```python
from build123d import *

# Parameters (mm, degrees)
BOSS_EXTRUDE1_DEPTH = 16.6624
CUT_EXTRUDE1_REACH  = 42.603
SKETCH5_R           = 4.1656
CUT_EXTRUDE2_REACH  = 42.603
SKETCH6_R           = 4.1656
CUT_EXTRUDE9_REACH  = 47.74
SKETCH27_R          = 9.525
CUT_EXTRUDE10_REACH = 47.74
SKETCH28_R          = 9.525


with BuildPart() as part:
    # Sketch4 → Boss-Extrude1 (new, symmetric)
    with BuildSketch(Plane(origin=(0, 0, 0), x_dir=(0, 0, -1), z_dir=(1, 0, 0))):
        with BuildLine():
            Line((-19.05, -19.05), (19.05, -19.05))
            Line((19.05, -19.05), (19.05, 19.05))
            Line((19.05, 19.05), (15.330256, 19.05))
            ThreePointArc((15.330256, 19.05), (12.900216, 18.566635), (10.840128, 17.190128))
            Line((10.840128, 17.190128), (-17.190128, -10.840128))
            ThreePointArc((-17.190128, -10.840128), (-18.566635, -12.900216), (-19.05, -15.330256))
            Line((-19.05, -15.330256), (-19.05, -19.05))
        make_face()
        Polygon((-10.069744, -12.7), (12.7, -12.7), (12.7, 10.069744), align=None, mode=Mode.SUBTRACT)
    extrude(amount=BOSS_EXTRUDE1_DEPTH, both=True)

    # Sketch5 → Cut-Extrude1 (cut, up to next)
    with BuildSketch(Plane(origin=(0, -12.7, 0), x_dir=(1, 0, 0), z_dir=(0, 1, 0)), mode=Mode.PRIVATE) as cut_extrude1_sk1:
        with Locations(Location((0, 0, 0), (0, 0, 270))):
            Circle(SKETCH5_R)
    cut_extrude1_tool1 = extrude(cut_extrude1_sk1.sketch, amount=-CUT_EXTRUDE1_REACH, mode=Mode.PRIVATE) & part.part
    add(cut_extrude1_tool1.solids().sort_by_distance((0, -12.7, 0))[0], mode=Mode.SUBTRACT)

    # Sketch6 → Cut-Extrude2 (cut, up to next)
    with BuildSketch(Plane.XY.offset(-12.7), mode=Mode.PRIVATE) as cut_extrude2_sk1:
        Circle(SKETCH6_R)
    cut_extrude2_tool1 = extrude(cut_extrude2_sk1.sketch, amount=-CUT_EXTRUDE2_REACH, mode=Mode.PRIVATE) & part.part
    add(cut_extrude2_tool1.solids().sort_by_distance((0, 0, -12.7))[0], mode=Mode.SUBTRACT)

    # Cut-Extrude9: up to this plane
    cut_extrude9_end = Plane(origin=(16.6624, -12.7, 10.069744), z_dir=(0, -0.7071067811865474, -0.7071067811865477))
    # Sketch27 → Cut-Extrude9 (cut, up to the surface)
    with BuildSketch(Plane.XY.offset(19.05), mode=Mode.PRIVATE) as cut_extrude9_sk1:
        with Locations(Location((0, 0, 0), (0, 0, 270))):
            Circle(SKETCH27_R)
    cut_extrude9_tool1 = split(extrude(cut_extrude9_sk1.sketch, amount=-CUT_EXTRUDE9_REACH, mode=Mode.PRIVATE), bisect_by=cut_extrude9_end, keep=Keep.BOTH, mode=Mode.PRIVATE)
    add(cut_extrude9_tool1.solids().sort_by_distance((0, 0, 19.05))[0], mode=Mode.SUBTRACT)

    # Cut-Extrude10: up to this face of the body (flat: up to its plane)
    cut_extrude10_end = Plane(part.part.faces().sort_by_distance((-16.258791, -12.7, -1.315128))[0])
    # Sketch28 → Cut-Extrude10 (cut, up to the picked face)
    with BuildSketch(Plane(origin=(0, 19.05, 0), x_dir=(1, 0, 0), z_dir=(0, 1, 0)), mode=Mode.PRIVATE) as cut_extrude10_sk1:
        Circle(SKETCH28_R)
    cut_extrude10_tool1 = split(extrude(cut_extrude10_sk1.sketch, amount=-CUT_EXTRUDE10_REACH, mode=Mode.PRIVATE), bisect_by=cut_extrude10_end, keep=Keep.BOTH, mode=Mode.PRIVATE)
    add(cut_extrude10_tool1.solids().sort_by(Axis((0, 19.05, 0), (0, -1, 0)))[0], mode=Mode.SUBTRACT)


solid = part.part
```
Geometry check sheet. Reference: the model listing, model coordinates, mm. A direction names the side the tool comes from. Round coordinates to 2 decimals unless told otherwise and drop trailing zeros. Order: outer loops, then holes, each group sorted by start corner. A loop starts at its lowest first (then second) coordinate and runs counter-clockwise, first axis right, second up. Notation, with made-up numbers: (-14.75, -36.75) - (19.25, -36.75) arc R24 ccw to (19.25, -17.75) - close; hole circle Ø10 at (0.25, 5). An arc over 180 degrees is marked (long way). Use a Markdown table: item, result. Add a question column.
(1) Sectioned sample at C-C, the plane y = 2. Enter the section's corners in (x, z) (3 decimals), and give its area (3 significant figures).
(2) Sectioned sample at A-A, the plane x = -14. Enter the section's corners in (y, z), and give its area (3 significant figures).
(3) Material ranges on line 1 along Z through (x, y) = (-2.5, 6); line 2 along X through (y, z) = (9.5, -3.5), recorded low to high. Write a range as [from, to].
(4) Sectioned sample at B-B, the plane z = -8.5. Enter the section's corners in (x, y) (3 decimals).
(5) Depth check by flat-ended pin: pin 1 (5 mm diameter, centred on x = -0.5, y = 2.5, fed in from +Z); pin 2 (6 mm diameter, centred on x = 8.5, z = 0, fed in from +Y). Enter the tip coordinate at first touch or a pass-through.
(6) Sectioned sample at D-D, the plane x = 0. Enter the section's corners in (y, z) (3 decimals), and give its area (3 significant figures).
(7) Tool access check on faces 4 (the cylindrical face through (0.25, 9.81, -9.52)), 5 (the flat face through (4, -4, -12.7)), 6 (the cylindrical face through (-0.25, -9.52, 9.81)). Record the directions out of +Z, -Z, +X, -X, +Y, -Y that give a thin tool (end or side, any length) a straight path to the whole face; none if there is none.
(8) Release check for a two-part mould opening along Z. For faces 1 (the cylindrical face through (3.973, 1.251, -15.831)), 2 (the cylindrical face through (1.251, -15.831, 3.973)), 3 (the cylindrical face through (0.233, -12.868, 18.553)) record: pulls with the +Z half, pulls with the -Z half, needs draft (parallel to the pull), parting line crosses it, or undercut.
Answers below:
| question | item | result |
|---|---|---|
| 1 | outline | (-16.662, -19.05) - (-3.654, -19.05) - (-3.654, -12.7) - (-16.662, -12.7) - close; (-16.662, -4.63) - (-9.313, -4.63) - (-9.313, -2) arc R9.525 cw to (-9.313, 2) - (-9.313, 4.35) - (-16.662, 4.35) - close; (3.654, -19.05) - (16.662, -19.05) - (16.662, -12.7) - (3.654, -12.7) - close; (9.313, -4.63) - (16.662, -4.63) - (16.662, 4.35) - (9.313, 4.35) - (9.313, 2) arc R9.525 cw to (9.313, -2) - close |
| 1 | area | 296 mm² |
| 2 | outline | (-19.05, -19.05) - (19.05, -19.05) - (19.05, -15.33) arc R6.35 ccw to (17.19, -10.84) - (-10.84, 17.19) arc R6.35 ccw to (-15.33, 19.05) - (-19.05, 19.05) - close; hole (-12.7, -12.7) - (10.07, -12.7) - (-12.7, 10.07) - close |
| 2 | area | 687 mm² |
| 3 | line 1 | [-19.05, -12.7] |
| 3 | line 2 | [-16.66, -8.86], [8.86, 16.66] |
| 4 | outline | (-16.662, -19.05) - (16.662, -19.05) - (16.662, -12.7) - (-16.662, -12.7) - close; (-16.662, 5.87) - (-7.501, 5.87) arc R9.525 cw to (-4.298, 8.5) - (-4.298, 14.85) - (-16.662, 14.85) - close; (4.298, 8.5) arc R9.525 cw to (7.501, 5.87) - (16.662, 5.87) - (16.662, 14.85) - (4.298, 14.85) - close |
| 5 | pin 1 | z = -12.7 |
| 5 | pin 2 | y = 9.3 |
| 6 | outline | (-19.05, -19.05) - (-4.166, -19.05) - (-4.166, -12.7) - (-12.7, -12.7) - (-12.7, -4.166) - (-19.05, -4.166) - close; (-19.05, 4.166) - (-12.7, 4.166) - (-12.7, 10.07) - (-12.155, 9.525) - (-9.525, 9.525) - (-9.525, 15.875) - (-10.84, 17.19) arc R6.35 ccw to (-15.33, 19.05) - (-19.05, 19.05) - close; (4.166, -19.05) - (19.05, -19.05) - (19.05, -15.33) arc R6.35 ccw to (17.19, -10.84) - (15.875, -9.525) - (9.525, -9.525) - (9.525, -12.155) - (10.07, -12.7) - (4.166, -12.7) - close |
| 6 | area | 386 mm² |
| 7 | face 4 | +Y |
| 7 | face 5 | +X, -X |
| 7 | face 6 | +Z |
| 8 | face 1 | needs draft |
| 8 | face 2 | undercut |
| 8 | face 3 | pulls with the +Z half |
